Build history of the part. All positions in model axes, mm. A direction names the side the tool comes from. Coordinates: 2 decimals unless noted, no trailing zeros. Write each loop counter-clockwise with the first axis right and the second up, starting at its lowest first coordinate (ties: lowest second). Pieces come first, ordered by that corner, then holes. Notation, with made-up numbers: (-39.75, 11) -> (-24.75, 11) arc R21 cw to (-24.75, 33) -> close; hole circle Ø9 at (32, 3). An arc over 180 degrees is marked (long way). Write each question's results on one line, items separated by ' | '. Start each with the question number.
Q1. Drill centre lines: line 1 (X direction, y = -90.5, z = 2); line 2 (X direction, y = -81.5, z = -8); line 3 (Y direction, x = 25, z = 21). Where is each one in solid material? Low to high.
Q2. Saw through at A-A on y = -30. Give the cut face in (x, z), and give its area (3 significant figures).
Q3. Drop flat-ended pins along their axis: pin 1 Ø7.5 at (x, z) = (-177, 4.5) entering from -Y; pin 2 Ø1.5 at (x, z) = (103, 23.5) entering from -Y; pin 3 Ø4 at (x, y) = (-3, -10) entering from -Z; pin 4 Ø6 at (y, z) = (-178, 31) entering from -X. Give the stop position or say it passes through.
Q4. Saw through at B-B on z = 12. Give the cut face in (x, y), and give its area (3 significant figures).
Q5. Saw through at C-C on y = -278.5. Give the cut face in (x, z).
Q6. Tool access for faces 1 (the face through (172, -176, -15)), 2 (the face through (14, -14, 26)), 3 (the face through (0, -10, 0)), 4 (the face through (-172, -179, -13)), 5 (the face through (175, -354, -5)): list every direction of +Z, -Z, +X, -X, +Y, -Y with a clear straight run to the whole face (end or side of a thin tool).
Q7. Saw through at D-D on x = -113. Give the cut face in (y, z), and give its area (3 significant figures).
from build123d import *

# Parameters (mm, degrees)
EXTRUDE_1_DEPTH        = 26
EXTRUDE_2_DEPTH        = 19
FILLET_1_R             = 10
SKETCH_5_W             = 161
SKETCH_5_H             = 6
CUT_EXTRUDE_1_DEPTH    = 52
SKETCH_1_5_W           = 11
SKETCH_1_5_H           = 340
EXTRUDE_4_DEPTH        = 7
SKETCH_6_W             = 1.9
SKETCH_6_H             = 2
SKETCH_6_W_2           = 6.6
EXTRUDE_5_DEPTH        = 28
SKETCH_6_3_W           = 6.6
SKETCH_6_3_H           = 2
CUT_EXTRUDE_2_DEPTH    = 5
FILLET_2_R             = 20
SKETCH_6_4_W           = 15
SKETCH_6_4_H           = 10
SKETCH_6_4_H_2         = 9
EXTRUDE_6_DEPTH        = 30
SKETCH_6_5_W           = 15
SKETCH_6_5_H           = 9
EXTRUDE_7_DEPTH        = 28
EXTRUDE_8_DEPTH        = 15
FILLET_3_R             = 20
FILLET_3_OF_MIRROR_2_R = 20
FILLET_4_R             = 20


with BuildPart() as part:
    # 스케치1 → 보스-돌출1 (new body)
    with BuildSketch(Plane.XY):
        Polygon((-168, 0), (168, 0), (183, 0), (183, -340), (168, -340), (168, -20), (-168, -20), (-168, -340), (-183, -340), (-183, 0), align=None)
    extrude(amount=EXTRUDE_1_DEPTH)

    # 스케치1<4> → 보스-돌출2 (add)
    with BuildSketch(Plane.XY):
        Polygon((172, 0), (168, 0), (168, -20), (168, -340), (172, -340), align=None)
        Polygon((-168, -20), (-168, 0), (-172, 0), (-172, -340), (-168, -340), align=None)
    extrude(amount=-EXTRUDE_2_DEPTH)

    # 필렛1
    fillet_1_edges = [part.edges().sort_by_distance(p)[0] for p in [
        (170, 0, -19),
        (170, -340, -19),
        (-170, -340, -19),
        (-170, 0, -19),
    ]]
    fillet(fillet_1_edges, radius=FILLET_1_R)

    # 스케치5 → 컷-돌출1 (cut)
    with BuildSketch(Plane(origin=(0, 0, 0), x_dir=(1, 0, 0), z_dir=(0, 1, 0))):
        with Locations((-87.5, -3)):
            Rectangle(SKETCH_5_W, SKETCH_5_H)
        with Locations((87.5, -3)):
            Rectangle(SKETCH_5_W, SKETCH_5_H)
    extrude(amount=-CUT_EXTRUDE_1_DEPTH, mode=Mode.SUBTRACT)

    # 스케치1<5> → 보스-돌출4 (add)
    with BuildSketch(Plane.XY):
        with Locations((177.5, -170)):
            Rectangle(SKETCH_1_5_W, SKETCH_1_5_H)
        with Locations((-177.5, -170)):
            Rectangle(SKETCH_1_5_W, SKETCH_1_5_H)
    extrude(amount=-EXTRUDE_4_DEPTH)

    # 스케치6 → 보스-돌출5 (add)
    with BuildSketch(Plane.XZ.offset(340)):
        with Locations((-182.05, -6)):
            Rectangle(SKETCH_6_W, SKETCH_6_H)
        with Locations((-177.8, -6)):
            Rectangle(SKETCH_6_W_2, SKETCH_6_H)
        Polygon((-174.5, -7), (-172, -7), (-168, -7), (-168, -5), (-174.5, -5), align=None)
    extrude_5 = extrude(amount=EXTRUDE_5_DEPTH)

    # 스케치6<3> → 컷-돌출2 (cut)
    with BuildSketch(Plane.XZ.offset(340)):
        with Locations((-177.8, -6)):
            Rectangle(SKETCH_6_3_W, SKETCH_6_3_H)
    cut_extrude_2 = extrude(amount=CUT_EXTRUDE_2_DEPTH, mode=Mode.SUBTRACT)

    # 필렛2
    # the kernel refuses this fillet: 20 mm, written as the material it adds along each edge
    with BuildSketch(Plane(origin=(-172, -340, -7), x_dir=(0, -1, 0), z_dir=(1, 0, 0))) as fillet_2_piece_1:
        with BuildLine():
            CenterArc((14, 20), FILLET_2_R, 216.869897646, 53.130102354)
            Line((-2, 8), (-3.6, 6.8))
            ThreePointArc((-3.6, 6.8), (-2, 2), (-2, 0))
            Line((-2, 0), (0, -2))
            Line((0, -2), (14, -2))
            Line((14, -2), (14, 0))
        make_face()
    extrude(amount=4)

    # 스케치6<4> → 보스-돌출6 (add)
    with BuildSketch(Plane.XZ.offset(340)):
        with Locations((-175.5, 31)):
            Rectangle(SKETCH_6_4_W, SKETCH_6_4_H)
        with Locations((-175.5, 40.5)):
            Rectangle(SKETCH_6_4_W, SKETCH_6_4_H_2)
    extrude_6 = extrude(amount=-EXTRUDE_6_DEPTH)

    # 스케치6<5> → 보스-돌출7 (add)
    with BuildSketch(Plane.XZ.offset(340)):
        with Locations((-175.5, 40.5)):
            Rectangle(SKETCH_6_5_W, SKETCH_6_5_H)
    extrude_7 = extrude(amount=EXTRUDE_7_DEPTH)

    # 스케치9 → 보스-돌출8 (add)
    with BuildSketch(Plane.ZY.offset(183)):
        Polygon((26, -310), (45, -310), (26, -270), align=None)
    extrude_8 = extrude(amount=-EXTRUDE_8_DEPTH)

    # 필렛3
    fillet_3_edges = [part.edges().sort_by_distance(p)[0] for p in [
        (-175.5, -310, 45),
        (-175.5, -270, 26),
    ]]
    fillet(fillet_3_edges, radius=FILLET_3_R)

    # 대칭 복사2: 보스-돌출5, 컷-돌출2, 보스-돌출6, 보스-돌출7, 보스-돌출8 across plane
    add(extrude_5.mirror(Plane(origin=(0, 0, 0), x_dir=(0, 0, 1), z_dir=(1, 0, 0))))
    add(cut_extrude_2.mirror(Plane(origin=(0, 0, 0), x_dir=(0, 0, 1), z_dir=(1, 0, 0))), mode=Mode.SUBTRACT)
    add(extrude_6.mirror(Plane(origin=(0, 0, 0), x_dir=(0, 0, 1), z_dir=(1, 0, 0))))
    add(extrude_7.mirror(Plane(origin=(0, 0, 0), x_dir=(0, 0, 1), z_dir=(1, 0, 0))))
    add(extrude_8.mirror(Plane(origin=(0, 0, 0), x_dir=(0, 0, 1), z_dir=(1, 0, 0))))

    # 필렛3 of 대칭 복사2
    fillet_3_of_mirror_2_edges = [part.edges().sort_by_distance(p)[0] for p in [
        (175.5, -310, 45),
        (175.5, -270, 26),
    ]]
    fillet(fillet_3_of_mirror_2_edges, radius=FILLET_3_OF_MIRROR_2_R)

    # 필렛4
    # the kernel refuses this fillet: 20 mm, written as the material it adds along each edge
    with BuildSketch(Plane(origin=(172, -340, -7), x_dir=(0, 0.24253562503633938, -0.9701425001453302), z_dir=(-1, 0, 0))) as fillet_4_piece_1:
        with BuildLine():
            CenterArc((16.007351252, 18.432707503), FILLET_4_R, 194.036243468, 53.130102354)
            Line((-3.395498751, 13.581995002), (-5.335783751, 13.096923752))
            Line((-5.335783751, 13.096923752), (-1.940285, -0.48507125))
            Line((-1.940285, -0.48507125), (0.48507125, -1.940285))
            ThreePointArc((0.48507125, -1.940285), (2.42535625, -1.45521375), (7.470097251, -1.84327075))
            Line((7.470097251, -1.84327075), (8.246211251, 0))
        make_face()
    extrude(amount=4)


solid = part.part
Returned:
1) line 1: x = -183 to -168, 168 to 183 | line 2: x = -172 to -168, 168 to 172 | line 3: y = -20 to 0
2) outline: (-183, -7) -> (-172, -7) -> (-172, -19) -> (-168, -19) -> (-168, 26) -> (-183, 26) -> close; (168, -19) -> (172, -19) -> (172, -7) -> (183, -7) -> (183, 26) -> (168, 26) -> close | area: 1,090 mm2
3) pin 1: stops at y = -340 | pin 2: stops at y = -20 | pin 3: stops at z = 0 | pin 4: passes through
4) outline: (-183, -340) -> (-168, -340) -> (-168, -20) -> (168, -20) -> (168, -340) -> (183, -340) -> (183, 0) -> (-183, 0) -> close | area: 16,900 mm2
5) outline: (-183, -7) -> (-172, -7) -> (-172, -19) -> (-168, -19) -> (-168, 30.04) -> (-183, 30.04) -> close; (168, -19) -> (172, -19) -> (172, -7) -> (183, -7) -> (183, 30.04) -> (168, 30.04) -> close
6) face 1: -Z, +X, +Y, -Y | face 2: +Z, +X, -X, +Y | face 3: -Z, +Y, -Y | face 4: -Z, -X, +Y, -Y | face 5: +X, -X, -Y
7) outline: (-20, 6) -> (0, 6) -> (0, 26) -> (-20, 26) -> close | area: 400 mm2
